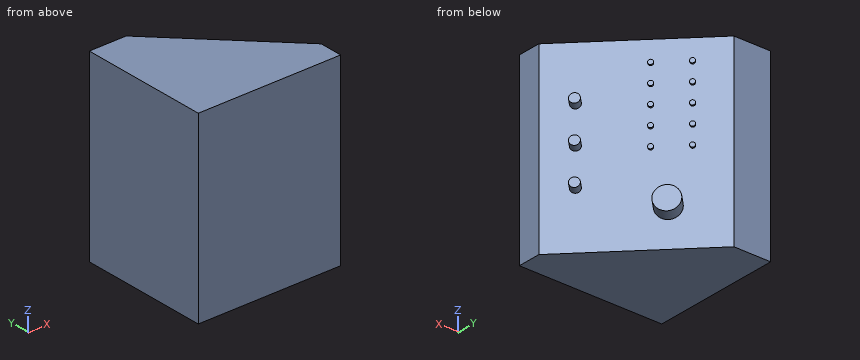
Autodesk Inventor part; units mm, degrees
ref_plane "YZ Plane" through (0, 0, 0) normal (1, 0, 0) x (0, 1, 0)
ref_plane "XZ Plane" through (0, 0, 0) normal (0, 1, 0) x (-1, 0, 0)
ref_plane "XY Plane" through (0, 0, 0) normal (0, 0, 1) x (1, 0, 0)
sketch "Sketch1" plane through (0, 0, 0) normal (0, 0, 1) x (1, 0, 0)
  line L0 (0, 0) -> (155, 0)
  line L1 (155, 0) -> (155, 25)
  line L2 (155, 25) -> (40, 140)
  line L3 (40, 140) -> (0, 140)
  line L4 (0, 140) -> (0, 0)
  dimension "d4" = 40
  dimension "d5" = 140
  dimension "d10" = 25
  dimension "d13" = 45
extrude "Extrusion1" add sketch "Sketch1" along normal blind 200
sketch "Sketch2" plane through (40, 140, 0) normal (0.7071, 0.7071, 0) x (-0.7071, 0.7071, 0)
  circle A0 centre (-34.3317, 177.5117) radius 2.5
  point P0 (-70.7107, 0)
  dimension "d9" = 5
extrude "Extrusion2" add sketch "Sketch2" along normal blind 2
pattern_linear "Rectangular Pattern1" count 5 spacing 20 along (0, 0, -1) count 2 spacing 35 along (0.7071, -0.7071, 0) of "Extrusion2"
sketch "Sketch3" plane through (40, 140, 0) normal (0.7071, 0.7071, 0) x (-0.7071, 0.7071, 0)
  circle A0 centre (-54.6677, 40.8266) radius 12.5
  point P0 (-70.7107, 0)
  dimension "d20" = 25
extrude "Extrusion3" add sketch "Sketch3" along normal blind 15
sketch "Sketch4" plane through (40, 140, 0) normal (0.7071, 0.7071, 0) x (-0.7071, 0.7071, 0)
  circle A0 centre (-132.1111, 141.7709) radius 5
  point P0 (-70.7107, 0)
  dimension "d23" = 10
extrude "Extrusion4" add sketch "Sketch4" along normal blind 10
pattern_linear "Rectangular Pattern2" count 3 spacing 40 along (0, 0, -1) of "Extrusion4"
properties part number "genral outlines"
Here's how the part is built. I have some questions about the finished solid (model axes, mm). Give positions to 0.01 mm unless a question says otherwise; leave off trailing zeros. Order: outer loops, then holes, each group sorted by start corner. A loop starts at its lowest first (then second) coordinate and runs counter-clockwise, first axis right, second up. Notation, with made-up numbers: M -4,42 L 31,42 A13 ccw 31,50 Z; hole C 82,63.5 d6. An arc over 180 degrees is marked long. Answer as a JSON object with one key per item and string values. Group by question number.
1) Suppose I cut it at A-A, the plane z = 78.5. Write out the boundary of the cut face in (x, y), plus the area to 3 significant figures.
2) I'm going to push flat-ended pins straight in: pin 1 Ø1 at (x, y) = (110, 32.5) entering from -Z; pin 2 Ø4 at (y, z) = (57.5, 97) entering from +X. Where does each tip first touch, or does it pass through?
3) Please list where these lines run through material, in increasing order: L1, parallel to Y at x = 96.5, z = 45.5; L2, parallel to Y at x = 89, z = 10.5; L3, parallel to X at y = 86, z = 78. Write a range as [from, to].
4) Suppose I cut it at C-C, the plane x = 44. Write out the boundary of the cut face in (y, z), plus the area to 3 significant figures.
5) Suppose I cut it at D-D, the plane y = 53. Count the separate pieces of the cut face and the enclosed holes in it, plus the area to 3 significant figures.
6) Suppose I cut it at B-B, the plane y = 84. Write out the boundary of the cut face in (x, z), plus the area to 3 significant figures.
Results found:
{
 "1": {"outline": "M 0,0 L 155,0 L 155,25 L 40,140 L 0,140 Z", "area": "15,100 mm²"},
 "2": {"pin 1": "z = 0", "pin 2": "x = 138.55"},
 "3": {"L1": "[0, 83.5], [102.79, 104.71]", "L2": "[0, 91]", "L3": "[0, 94]"},
 "4": {"outline": "M 0,0 L 136,0 L 136,200 L 0,200 Z", "area": "27,200 mm²"},
 "5": {"separate pieces": "4", "enclosed holes": "0", "area": "25,600 mm²"},
 "6": {"outline": "M 0,0 L 96,0 L 96,200 L 0,200 Z", "area": "19,200 mm²"}
}
